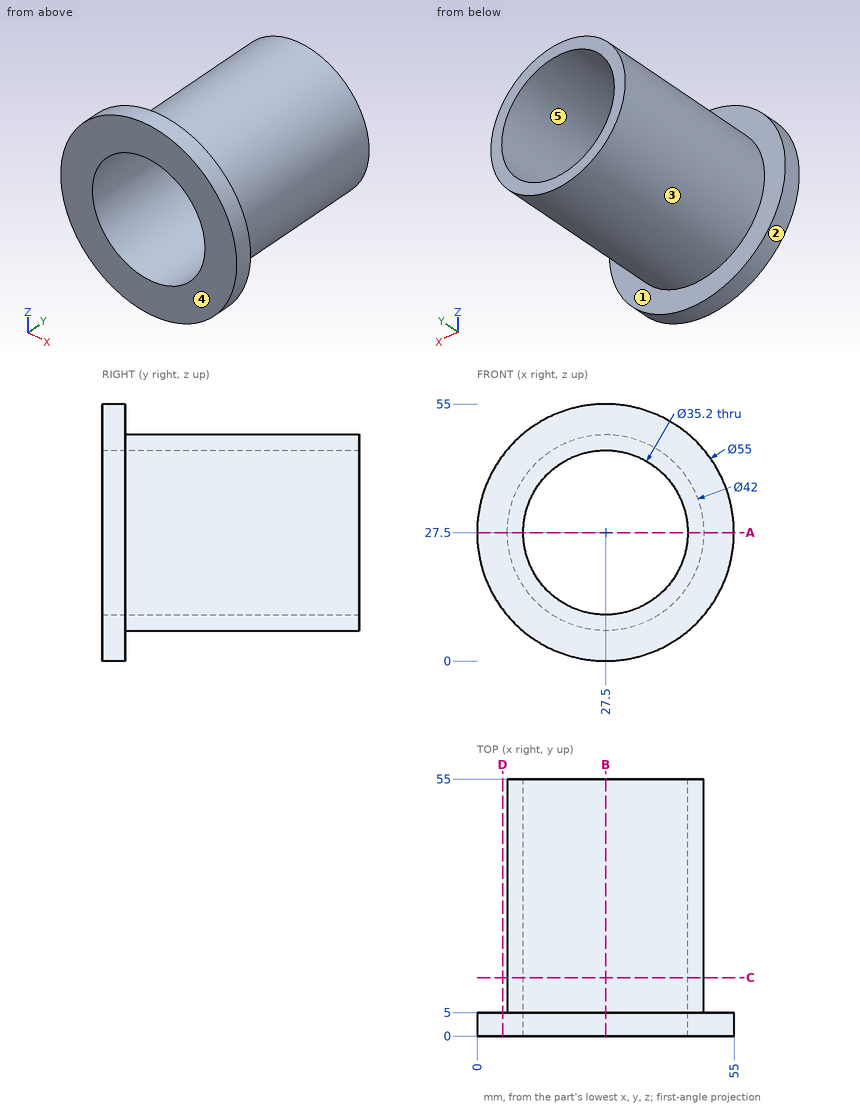
Study the drawing (mm; zero at the part's minimum x, y, z) and answer. A direction names the side the tool comes from. Give positions to 0.01 mm unless a question says otherwise; leave off trailing zeros. Write each loop counter-clockwise with the first axis right and the second up, starting at its lowest first coordinate (ties: lowest second). Pieces come first, ordered by that corner, then holes. Notation, with made-up numbers: (-36.5, 61) -> (-28.5, 61) arc R31 cw to (-28.5, 87) -> close; hole circle Ø6 at (-25.5, 70). An arc over 180 degrees is marked (long way). Answer in a Markdown table with one row per item.
1) Section D-D on x = 5.5 is taken. Give the vertices of the cut face in (y, z), plus the area to 3 significant figures.
Results list:
| item | result |
|---|---|
| outline | (0, 11) -> (5, 11) -> (5, 44) -> (0, 44) -> close |
| area | 165 mm^2 |
2) Section B-B on x = 27.5 is taken. Give the vertices of the cut face in (y, z), plus the area to 3 significant figures.
Results list:
| item | result |
|---|---|
| outline | (0, 0) -> (5, 0) -> (5, 6.5) -> (55, 6.5) -> (55, 9.9) -> (0, 9.9) -> close; (0, 45.1) -> (55, 45.1) -> (55, 48.5) -> (5, 48.5) -> (5, 55) -> (0, 55) -> close |
| area | 439 mm^2 |
3) Determine the mould class of the marked faces 3, 4 and 5 for opening direction X: released by +X, released by -X, zero draft, split by the parting line, or undercut.
Results list:
| item | result |
|---|---|
| face 3 | split by the parting line |
| face 4 | zero draft |
| face 5 | undercut |
4) Each of these flat-tipped pins is pushed along its axis until it touches: pin 1 Ø8 at (y, z) = (23, 24) entering from +X; pin 2 Ø8 at (x, y) = (42.5, 48.5) entering from -Z; pin 3 Ø10 at (x, y) = (14.5, 40.5) entering from +Z. Where does it stop, or does it pass through?
Results list:
| item | result |
|---|---|
| pin 1 | x = 48.5 |
| pin 2 | z = 9.61 |
| pin 3 | z = 46.92 |
5) Straight lines are drawn through the part: line 1 (Z direction, x = 27.5, y = 43.5); line 2 (X direction, y = 25, z = 27); line 3 (Y direction, x = 41, z = 44). For each, find the intervals that lie inside material, in ascending order. Write a range as [from, to].
Results list:
| item | result |
|---|---|
| line 1 | [6.5, 9.9], [45.1, 48.5] |
| line 2 | [6.51, 9.91], [45.09, 48.49] |
| line 3 | [0, 5] |
6) Section C-C on y = 12.5 is taken. Give the vertices of the cut face in (x, z).
Results list:
| item | result |
|---|---|
| outline | circle Ø42 at (27.5, 27.5); hole circle Ø35.2 at (27.5, 27.5) |
7) A tool of negligible diameter and unlimited length cuts with its end or side. For the marked faces 1 and 2, from which of +Z, -Z, +X, -X, +Y, -Y can it reach the whole face along a straight path? Write none if from no direction.
Results list:
| item | result |
|---|---|
| face 1 | +Y |
| face 2 | +Y, -Y |
8) Section A-A on z = 27.5 is taken. Give the vertices of the cut face in (x, y), plus the area to 3 significant figures.
Results list:
| item | result |
|---|---|
| outline | (0, 0) -> (9.9, 0) -> (9.9, 55) -> (6.5, 55) -> (6.5, 5) -> (0, 5) -> close; (45.1, 0) -> (55, 0) -> (55, 5) -> (48.5, 5) -> (48.5, 55) -> (45.1, 55) -> close |
| area | 439 mm^2 |
